Read the model definition and answer for the solid it produces. Units are mm, in the model's axes. Give positions to 0.01 mm unless a question says otherwise; leave off trailing zeros. Order: outer loops, then holes, each group sorted by start corner. A loop starts at its lowest first (then second) coordinate and runs counter-clockwise, first axis right, second up.
Item 1: The mould has two halves that part along Y. Classify faces 1 (the face through (-1, -35, 2)), 2 (the face through (54.773, 30.358, 2.465)), 3 (the face through (0, -2, 5)): +Y half, -Y half, draft (parallel to the pull), parting line (faces both ways), or undercut.
Item 2: A cutting plane is placed at A-A (z = 1.5). Write down the section's boundary in (x, y).
Item 3: A cutting plane is placed at C-C (y = -14). Write down the section's boundary in (x, z).
Item 4: A cutting plane is placed at B-B (x = -34). Write down the section's boundary in (y, z).
Item 5: A cutting plane is placed at D-D (y = 30). Write down the section's boundary in (x, z), plus the area to 3 significant figures.
Item 6: Find the intervals of material crossed by line 1 along Y through (x, z) = (-57.5, 3.8); line 2 along Y through (x, z) = (34, 3.75); line 3 along X through (y, z) = (-13.5, 0.6), in increasing order.
Autodesk Inventor part; units mm, degrees
ref_plane "YZ Plane" through (0, 0, 0) normal (1, 0, 0) x (0, 1, 0)
ref_plane "XZ Plane" through (0, 0, 0) normal (0, 1, 0) x (-1, 0, 0)
ref_plane "XY Plane" through (0, 0, 0) normal (0, 0, 1) x (1, 0, 0)
sketch "Sketch1" plane through (0, 0, 0) normal (0, 0, 1) x (1, 0, 0)
  line L0 (-70, -35) -> (70, -35)
  line L1 (70, -35) -> (70, 35)
  line L2 (70, 35) -> (-70, 35)
  line L3 (-70, 35) -> (-70, -35)
  line L4 (-70, -35) -> (70, 35) construction
  line L5 (70, -35) -> (-70, 35) construction
  point P0 (0, 0)
  dimension "d0" = 140
  dimension "d1" = 70
extrude "Extrusion1" add sketch "Sketch1" along normal blind 5
sketch "Sketch2" plane through (0, 0, 5) normal (0, 0, 1) x (1, 0, 0)
  line L0 (-57.5, -30) -> (57.5, -30) construction
  line L1 (57.5, -30) -> (57.5, 30) construction
  line L2 (57.5, 30) -> (-57.5, 30) construction
  line L3 (-57.5, 30) -> (-57.5, -30) construction
  line L4 (-57.5, -30) -> (57.5, 30) construction
  line L5 (57.5, -30) -> (-57.5, 30) construction
  point P0 (0, 0)
  dimension "d4" = 115
  dimension "d5" = 60
hole "Hole1" at (-57.5, -30, 5) at (-57.5, 30, 5) at (57.5, 30, 5) at (57.5, -30, 5) direction (0, 0, -1) diameter 5.5 depth 8 tip angle 118
fillet "Fillet1" radius 2 4 edges at (70, 35, 2.5) (70, -35, 2.5) (-70, 35, 2.5) (-70, -35, 2.5)
sketch "Sketch3" plane through (0, 0, 5) normal (0, 0, 1) x (1, 0, 0)
  circle A0 centre (-34, 0) radius 32
  circle A1 centre (34, 0) radius 32
  line L0 (-34, 0) -> (34, 0) construction
  point P0 (0, 0)
  point P1 (0, 0)
  dimension "d14" = 64
  dimension "d15" = 64
  dimension "d16" = 68
extrude "Extrusion2" cut sketch "Sketch3" against normal blind 5
properties part number "MidStück_Caps" material "Polycarbonate, Clear"
Response values:
1. face 1: -Y half
1. face 2: undercut
1. face 3: draft
2. outline: (-70, -33) arc R2 ccw to (-68, -35) - (68, -35) arc R2 ccw to (70, -33) - (70, 33) arc R2 ccw to (68, 35) - (-68, 35) arc R2 ccw to (-70, 33) - close; hole circle Ø64 at (-34, 0); hole circle Ø5.5 at (-57.5, -30); hole circle Ø5.5 at (-57.5, 30); hole circle Ø64 at (34, 0); hole circle Ø5.5 at (57.5, -30); hole circle Ø5.5 at (57.5, 30)
3. outline: (-70, 0) - (-62.77, 0) - (-62.77, 5) - (-70, 5) - close; (-5.23, 0) - (5.23, 0) - (5.23, 5) - (-5.23, 5) - close; (62.77, 0) - (70, 0) - (70, 5) - (62.77, 5) - close
4. outline: (-35, 0) - (-32, 0) - (-32, 5) - (-35, 5) - close; (32, 0) - (35, 0) - (35, 5) - (32, 5) - close
5. outline: (-70, 0) - (-60.25, 0) - (-60.25, 5) - (-70, 5) - close; (-54.75, 0) - (-45.14, 0) - (-45.14, 5) - (-54.75, 5) - close; (-22.86, 0) - (22.86, 0) - (22.86, 5) - (-22.86, 5) - close; (45.14, 0) - (54.75, 0) - (54.75, 5) - (45.14, 5) - close; (60.25, 0) - (70, 0) - (70, 5) - (60.25, 5) - close
5. area: 422 mm2
6. line 1: y = -35 to -32.75, -27.25 to -21.72, 21.72 to 27.25, 32.75 to 35
6. line 2: y = -35 to -32, 32 to 35
6. line 3: x = -70 to -63.01, -4.99 to 4.99, 63.01 to 70
